Input: part model. Units: mm. Frame: model coordinates. Round coordinates to 2 decimals unless told otherwise and drop trailing zeros. Loops run counter-clockwise (first coordinate to the right, second up) from the corner with the lowest first, then second, coordinate; pieces in that order, holes last. Notation, with made-up numbers: (71.5, 49.5) -> (113.5, 49.5) arc R18 ccw to (113.5, 53.5) -> close; hole circle Ø7 at (4.5, 43). An arc over 180 degrees is marked (long way). Answer as a JSON object with one key per item and string values.
```python
from build123d import *

# Parameters (mm, degrees)
PAD004_DEPTH    = 2.5
SKETCH011_R     = 1
POCKET002_DEPTH = 3
FILLET_R        = 0.5


with BuildPart() as part:
    # Sketch006 → Pad004 (new body)
    with BuildSketch(Plane(origin=(43, -2, 9), x_dir=(1, 0, 0), z_dir=(0, 1, 0))):
        with BuildLine():
            Line((71.624302, 34.297205), (57.4953, 23.139806))
            ThreePointArc((57.4953, 23.139806), (56.374461, 21.744531), (55.974277, 20.000133))
            Line((55.974277, 20.000133), (55.975425, 9.975673))
            ThreePointArc((55.975425, 9.975673), (57.363966, 6.946234), (60.565113, 6.019837))
            Line((60.565113, 6.019837), (76.707381, 8.42585))
            Line((76.707381, 8.42585), (71.624302, 34.297205))
        make_face()
    extrude(amount=PAD004_DEPTH)

    # Sketch011 → Pocket002 (cut)
    with BuildSketch(Plane(origin=(43, 0.5, 9), x_dir=(1, 0, 0), z_dir=(0, 1, 0))):
        with Locations((60, 20)):
            Circle(SKETCH011_R)
        with Locations((60, 10)):
            Circle(SKETCH011_R)
    extrude(amount=-POCKET002_DEPTH, mode=Mode.SUBTRACT)

    # Fillet
    fillet_edges = [part.edges().sort_by_distance(p)[0] for p in [
        (107.559801, 0.5, -19.718506),
        (117.165842, 0.5, -12.361528),
        (99.374461, 0.5, -12.744531),
        (111.636247, 0.5, 1.777156),
        (98.974851, 0.5, -5.987903),
        (100.363966, 0.5, 2.053766),
        (102, 0.5, -1),
        (102, 0.5, -11),
    ]]
    fillet(fillet_edges, radius=FILLET_R)


solid = part.part
```
1) Section B-B, the plane x = 103. Count the separate pieces of the cut face and the enclosed holes in it, plus the area to 3 significant figures.
Output:
{"separate pieces": "3", "enclosed holes": "0", "area": "37.5 mm^2"}
2) Contact query for flat-ended pins moving along their axis: P1, Ø10, axis at x = 102.5, z = -20.5, coming from the -Y side; P2, Ø2.5, axis at x = 103, z = -1, coming from the +Y side. Output: stop coordinate, or through.
Output:
{"P1": "stops at y = -2", "P2": "stops at y = 0.43"}
3) Ray query, probe 1 along Z at (x, y) = (103, -0.55); probe 2 along X at (y, z) = (-0.6, -11); probe 3 along X at (y, z) = (-0.3, -11.5). Return the intervals inside material, ascending.
Output:
{"probe 1": "z = -16.12 to -12, -10 to -2, 0 to 3.02", "probe 2": "x = 98.97 to 102, 104 to 117.43", "probe 3": "x = 99.01 to 102.13, 103.87 to 117.34"}
4) Section A-A, the plane y = -1.1. Output: boundary loops of the cut face in (x, z), plus the area to 3 significant figures.
Output:
{"outline": "(98.97, -11) arc R4 ccw to (100.5, -14.14) -> (114.62, -25.3) -> (119.71, 0.57) -> (103.57, 2.98) arc R4 ccw to (98.98, -0.98) -> close; hole circle Ø2 at (103, -11); hole circle Ø2 at (103, -1)", "area": "394 mm^2"}
5) Draft query along Z for faces 1 (the face through (111.73, 0.35, 1.62)), 2 (the face through (107.55, 0.35, -19.53)), 3 (the face through (102, -1, -1)). Return one class per face: +Z half, -Z half, draft (parallel to the pull), parting line (faces both ways), or undercut.
Output:
{"face 1": "+Z half", "face 2": "-Z half", "face 3": "undercut"}
